```python
from build123d import *

# Parameters (mm, degrees)
SKETCH_1_W          = 20
SKETCH_1_H          = 510
SKETCH_1_R          = 1.5
EXTRUDE_1_DEPTH     = 3
SKETCH_2_W          = 20
SKETCH_2_H          = 20
CUT_EXTRUDE_1_DEPTH = 257.099704345
FILLET_1_R          = 3
SKETCH_3_R          = 1.5
CUT_EXTRUDE_2_DEPTH = 255.347452337


with BuildPart() as part:
    # 草图1 → 凸台-拉伸1 (new body)
    with BuildSketch(Plane(origin=(0, 0, 0), x_dir=(1, 0, 0), z_dir=(0, 1, 0))):
        with Locations((0.250541192, -0.876894172)):
            Rectangle(SKETCH_1_W, SKETCH_1_H)
        with Locations(Location((5.250541192, -103.876894172, 0), (0, 0, 270))):
            Circle(SKETCH_1_R, mode=Mode.SUBTRACT)
        with Locations(Location((-4.749458808, -103.876894172, 0), (0, 0, 270))):
            Circle(SKETCH_1_R, mode=Mode.SUBTRACT)
        with Locations(Location((6.213384437, -46.87688957, 0), (0, 0, 270))):
            Circle(SKETCH_1_R, mode=Mode.SUBTRACT)
        with Locations(Location((-5.786615563, -46.87688957, 0), (0, 0, 270))):
            Circle(SKETCH_1_R, mode=Mode.SUBTRACT)
        with Locations(Location((6.213384437, -24.87688957, 0), (0, 0, 270))):
            Circle(SKETCH_1_R, mode=Mode.SUBTRACT)
        with Locations(Location((-5.786615563, -24.87688957, 0), (0, 0, 270))):
            Circle(SKETCH_1_R, mode=Mode.SUBTRACT)
        with Locations(Location((6.295138669, 53.123077011, 0), (0, 0, 270))):
            Circle(SKETCH_1_R, mode=Mode.SUBTRACT)
        with Locations(Location((-5.704861331, 53.123077011, 0), (0, 0, 270))):
            Circle(SKETCH_1_R, mode=Mode.SUBTRACT)
        with Locations(Location((6.295138669, 75.123077011, 0), (0, 0, 270))):
            Circle(SKETCH_1_R, mode=Mode.SUBTRACT)
        with Locations(Location((-5.704861331, 75.123077011, 0), (0, 0, 270))):
            Circle(SKETCH_1_R, mode=Mode.SUBTRACT)
        with Locations(Location((6.263384437, 84.37311043, 0), (0, 0, 270))):
            Circle(SKETCH_1_R, mode=Mode.SUBTRACT)
        with Locations(Location((-5.736615563, 84.37311043, 0), (0, 0, 270))):
            Circle(SKETCH_1_R, mode=Mode.SUBTRACT)
        with Locations(Location((6.263384437, 94.37311043, 0), (0, 0, 270))):
            Circle(SKETCH_1_R, mode=Mode.SUBTRACT)
        with Locations(Location((-5.736615563, 94.37311043, 0), (0, 0, 270))):
            Circle(SKETCH_1_R, mode=Mode.SUBTRACT)
        with Locations(Location((6.250541192, 103.123105828, 0), (0, 0, 270))):
            Circle(SKETCH_1_R, mode=Mode.SUBTRACT)
        with Locations(Location((-5.749458808, 103.123105828, 0), (0, 0, 270))):
            Circle(SKETCH_1_R, mode=Mode.SUBTRACT)
        with Locations(Location((6.250541192, 125.123105828, 0), (0, 0, 270))):
            Circle(SKETCH_1_R, mode=Mode.SUBTRACT)
        with Locations(Location((-5.749458808, 125.123105828, 0), (0, 0, 270))):
            Circle(SKETCH_1_R, mode=Mode.SUBTRACT)
        with Locations(Location((6.345138669, 184.373077011, 0), (0, 0, 270))):
            Circle(SKETCH_1_R, mode=Mode.SUBTRACT)
        with Locations(Location((-5.654861331, 184.373077011, 0), (0, 0, 270))):
            Circle(SKETCH_1_R, mode=Mode.SUBTRACT)
        with Locations(Location((6.345138669, 194.373077011, 0), (0, 0, 270))):
            Circle(SKETCH_1_R, mode=Mode.SUBTRACT)
        with Locations(Location((-5.654861331, 194.373077011, 0), (0, 0, 270))):
            Circle(SKETCH_1_R, mode=Mode.SUBTRACT)
        with Locations(Location((6.300541192, 234.373105828, 0), (0, 0, 270))):
            Circle(SKETCH_1_R, mode=Mode.SUBTRACT)
        with Locations(Location((-5.699458808, 234.373105828, 0), (0, 0, 270))):
            Circle(SKETCH_1_R, mode=Mode.SUBTRACT)
        with Locations(Location((6.300541192, 244.373105828, 0), (0, 0, 270))):
            Circle(SKETCH_1_R, mode=Mode.SUBTRACT)
        with Locations(Location((-5.699458808, 244.373105828, 0), (0, 0, 270))):
            Circle(SKETCH_1_R, mode=Mode.SUBTRACT)
    extrude(amount=EXTRUDE_1_DEPTH)

    # 草图2 → 切除-拉伸1 (cut, through all)
    with BuildSketch(Plane(origin=(0, 3, 0), x_dir=(1, 0, 0), z_dir=(0, 1, 0))):
        with Locations((0.250541192, -245.876894172)):
            Rectangle(SKETCH_2_W, SKETCH_2_H)
    extrude(amount=-CUT_EXTRUDE_1_DEPTH, mode=Mode.SUBTRACT)

    # 圆角1
    fillet_1_edges = [part.edges().sort_by_distance(p)[0] for p in [
        (-9.749458808, 1.5, 235.876894172),
        (10.250541192, 1.5, 235.876894172),
        (10.250541192, 1.5, -254.123105828),
        (-9.749458808, 1.5, -254.123105828),
    ]]
    fillet(fillet_1_edges, radius=FILLET_1_R)

    # 草图3 → 切除-拉伸2 (cut, through all)
    with BuildSketch(Plane(origin=(0, 3, 0), x_dir=(1, 0, 0), z_dir=(0, 1, 0))):
        with Locations(Location((-5.749458808, -170.876894172, 0), (0, 0, 270))):
            Circle(SKETCH_3_R)
        with Locations(Location((-5.749458808, -200.876894172, 0), (0, 0, 270))):
            Circle(SKETCH_3_R)
        with Locations(Location((6.250541192, -170.876894172, 0), (0, 0, 90))):
            Circle(SKETCH_3_R)
        with Locations(Location((6.250541192, -200.876894172, 0), (0, 0, 90))):
            Circle(SKETCH_3_R)
    extrude(amount=-CUT_EXTRUDE_2_DEPTH, mode=Mode.SUBTRACT)


solid = part.part
```
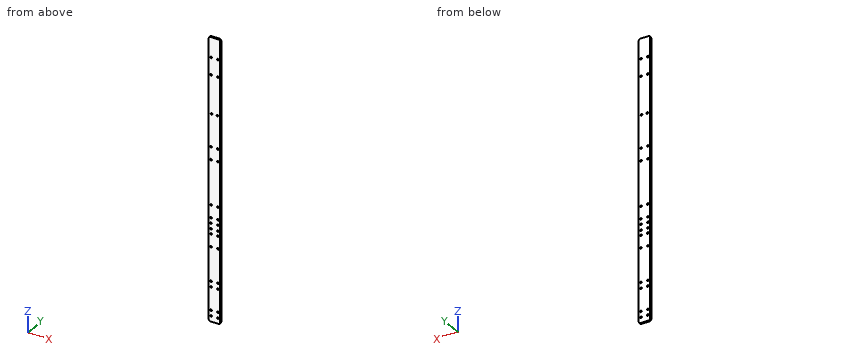
Design review of the part built by this model. Coordinates are the model's own, in mm. Round coordinates to 2 decimals unless told otherwise and drop trailing zeros.
Item 1: Clearance check with flat-ended pins moving along their axes: pin 1 Ø1 at (x, z) = (7, -81.5) entering from -Y; pin 2 Ø1.8 at (x, z) = (6.3, -75.12) entering from -Y. State where each tip first meets the part, or that it passes through.
Item 2: We need section A-A on y = 2.2. State how many separate pieces and enclosed holes the cut face has, and give its area (3 significant figures).
Item 3: For probe 1 along X at (y, z) = (1.4, 47.5); probe 2 along X at (y, z) = (0.75, -183); probe 3 along Z at (x, y) = (-7.5, 2.8), list the stretches that pass through material, from the lowest coordinate up.
Returned:
1. pin 1: stops at y = 0
1. pin 2: passes through
2. separate pieces: 1
2. enclosed holes: 30
2. area: 9,580 mm2
3. probe 1: x = -9.75 to -7.15, -4.42 to 4.85, 7.58 to 10.25
3. probe 2: x = -9.75 to -6.26, -5.05 to 5.74, 6.95 to 10.25
3. probe 3: z = -254.03 to 235.78
